Input: part model. Units: mm. Frame: model coordinates. Round coordinates to 2 decimals unless told otherwise and drop trailing zeros. Write each loop counter-clockwise with the first axis right and the second up, starting at its lowest first coordinate (ties: lowest second). Pieces come first, ordered by that corner, then holes. Notation, with made-up numbers: (-12.5, 56) - (43.5, 56) arc R23 ccw to (43.5, 70) - close; hole circle Ø9 at (7, 42.25). An arc over 180 degrees is marked (long way). Use one line per item in the form item = value.
```python
from build123d import *

# Parameters (mm, degrees)
F0_W     = 4.6228
F0_H     = 4.6228
F1_DEPTH = 1.27


with BuildPart() as f1:
    # F0 (on Top) → F1 (new body)
    with BuildSketch(Plane.XY):
        Polygon((78.031066, -39.672382), (78.031066, -1.572382), (73.992466, -1.572382), (73.992466, 1.602618), (69.369666, 1.602618), (69.369666, -1.572382), (61.292466, -1.572382), (61.292466, 1.602618), (56.669666, 1.602618), (56.669666, -1.572382), (48.592466, -1.572382), (48.592466, 1.602618), (43.969666, 1.602618), (43.969666, -1.572382), (35.892466, -1.572382), (35.892466, 1.602618), (31.269666, 1.602618), (31.269666, -1.572382), (23.192466, -1.572382), (23.192466, 1.602618), (18.569666, 1.602618), (18.569666, -1.572382), (10.492466, -1.572382), (10.492466, 1.602618), (5.869666, 1.602618), (5.869666, -1.572382), (-2.207534, -1.572382), (-2.207534, 1.602618), (-6.830334, 1.602618), (-6.830334, -1.572382), (-10.868934, -1.572382), (-10.868934, -33.322382), (-10.868934, -39.672382), (-6.830334, -39.672382), (-6.830334, -42.847382), (-2.207534, -42.847382), (-2.207534, -39.672382), (5.869666, -39.672382), (5.869666, -42.847382), (10.492466, -42.847382), (10.492466, -39.672382), (18.569666, -39.672382), (18.569666, -42.847382), (23.192466, -42.847382), (23.192466, -39.672382), (31.269666, -39.672382), (31.269666, -42.847382), (35.892466, -42.847382), (35.892466, -39.672382), (43.969666, -39.672382), (43.969666, -42.847382), (48.592466, -42.847382), (48.592466, -39.672382), (56.669666, -39.672382), (56.669666, -42.847382), (61.292466, -42.847382), (61.292466, -39.672382), (69.369666, -39.672382), (69.369666, -42.847382), (73.992466, -42.847382), (73.992466, -39.672382), align=None)
        with Locations((-4.518934, -33.322382)):
            Rectangle(F0_W, F0_H, mode=Mode.SUBTRACT)
        with Locations((8.181066, -33.322382)):
            Rectangle(F0_W, F0_H, mode=Mode.SUBTRACT)
        with Locations((20.881066, -33.322382)):
            Rectangle(F0_W, F0_H, mode=Mode.SUBTRACT)
        with Locations((33.581066, -33.322382)):
            Rectangle(F0_W, F0_H, mode=Mode.SUBTRACT)
        with Locations((46.281066, -33.322382)):
            Rectangle(F0_W, F0_H, mode=Mode.SUBTRACT)
        with Locations((58.981066, -33.322382)):
            Rectangle(F0_W, F0_H, mode=Mode.SUBTRACT)
        with Locations((71.681066, -33.322382)):
            Rectangle(F0_W, F0_H, mode=Mode.SUBTRACT)
        with Locations((-4.518934, -20.622382)):
            Rectangle(F0_W, F0_H, mode=Mode.SUBTRACT)
        with Locations((8.181066, -20.622382)):
            Rectangle(F0_W, F0_H, mode=Mode.SUBTRACT)
        with Locations((20.881066, -20.622382)):
            Rectangle(F0_W, F0_H, mode=Mode.SUBTRACT)
        with Locations((-4.518934, -7.922382)):
            Rectangle(F0_W, F0_H, mode=Mode.SUBTRACT)
        with Locations((8.181066, -7.922382)):
            Rectangle(F0_W, F0_H, mode=Mode.SUBTRACT)
        with Locations((20.881066, -7.922382)):
            Rectangle(F0_W, F0_H, mode=Mode.SUBTRACT)
        with Locations((33.581066, -20.622382)):
            Rectangle(F0_W, F0_H, mode=Mode.SUBTRACT)
        with Locations((46.281066, -20.622382)):
            Rectangle(F0_W, F0_H, mode=Mode.SUBTRACT)
        with Locations((58.981066, -20.622382)):
            Rectangle(F0_W, F0_H, mode=Mode.SUBTRACT)
        with Locations((71.681066, -20.622382)):
            Rectangle(F0_W, F0_H, mode=Mode.SUBTRACT)
        with Locations((33.581066, -7.922382)):
            Rectangle(F0_W, F0_H, mode=Mode.SUBTRACT)
        with Locations((46.281066, -7.922382)):
            Rectangle(F0_W, F0_H, mode=Mode.SUBTRACT)
        with Locations((58.981066, -7.922382)):
            Rectangle(F0_W, F0_H, mode=Mode.SUBTRACT)
        with Locations((71.681066, -7.922382)):
            Rectangle(F0_W, F0_H, mode=Mode.SUBTRACT)
    extrude(amount=F1_DEPTH)


solid = f1.part
```
(1) Material intervals for L1, parallel to Y at x = 48, z = 0.3; L2, parallel to Y at x = 50, z = 0.55, sorted ascending.
Derived:
L1 = -42.85 to -35.63, -31.01 to -22.93, -18.31 to -10.23, -5.61 to 1.6
L2 = -39.67 to -1.57
(2) Cut plane A-A on y = -9. Count the separate pieces of the cut face and the enclosed holes in it, then the cut area to 3 significant figures.
Derived:
separate_pieces = 8
enclosed_holes = 0
area = 71.8 mm^2
(3) Cut plane B-B on x = -3.5. Output: boundary loops of the cut face in (y, z), then the cut area to 3 significant figures.
Derived:
outline = (-42.85, 0) - (-35.63, 0) - (-35.63, 1.27) - (-42.85, 1.27) - close; (-31.01, 0) - (-22.93, 0) - (-22.93, 1.27) - (-31.01, 1.27) - close; (-18.31, 0) - (-10.23, 0) - (-10.23, 1.27) - (-18.31, 1.27) - close; (-5.61, 0) - (1.6, 0) - (1.6, 1.27) - (-5.61, 1.27) - close
area = 38.8 mm^2
(4) Cut plane D-D on x = 15.5. Output: boundary loops of the cut face in (y, z).
Derived:
outline = (-39.67, 0) - (-1.57, 0) - (-1.57, 1.27) - (-39.67, 1.27) - close
